Check sheet for the modelled part. Datum: model origin and axes. Units: mm. Face numbers are marked on the shaded views. A direction names the side the tool comes from. Round coordinates to 2 decimals unless told otherwise and drop trailing zeros. Write each loop counter-clockwise with the first axis right and the second up, starting at its lowest first coordinate (ties: lowest second). Pieces come first, ordered by that corner, then holes.
Item 1: Release check for a two-part mould opening along Y. For the marked faces 3, 4 and 5 record: +Y half, -Y half, draft (parallel to the pull), parting line (faces both ways), or undercut.
Item 2: Cross-section at C-C on x = 24. Enter the section's corners in (y, z), plus the area to 3 significant figures.
Item 3: Material ranges on line 1 (Z direction, x = 0, y = -1.7); line 2 (Y direction, x = 1, z = -26); line 3 (X direction, y = 11, z = -22.5), recorded low to high.
Item 4: Tool access check on the marked faces 1 and 2. Record the directions out of +Z, -Z, +X, -X, +Y, -Y that give a thin tool (end or side, any length) a straight path to the whole face; none if there is none.
Item 5: Cross-section at A-A on x = 0. Enter the section's corners in (y, z).
Item 6: Cross-section at D-D on z = -32.5. Enter the section's corners in (x, y).
Item 7: Cross-section at B-B on y = 13.5. Enter the section's corners in (x, z), plus the area to 3 significant figures.
Item 8: Go/stop test with flat-tipped pins: pin 1 Ø17.5 at (x, z) = (0, 0) entering from +Y; pin 2 Ø10 at (x, z) = (-9.5, 2) entering from +Y; pin 3 Ø8 at (x, y) = (-7.5, 16.5) entering from +Z; pin 4 Ø10 at (x, y) = (-20.5, 37.5) entering from +Z. Record where each tip stops, or that it passes through.
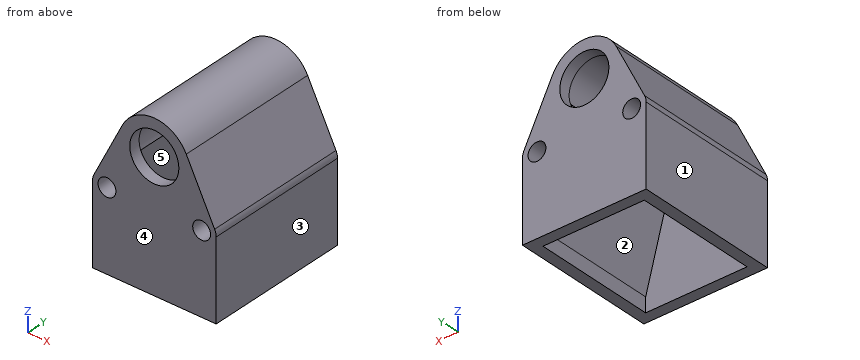
from build123d import *

# Parameters (mm, degrees)
SKETCH1_R           = 4
BOSS_EXTRUDE3_DEPTH = 55
SKETCH4_R           = 4
SKETCH4_R_2         = 11
BOSS_EXTRUDE4_DEPTH = 5
SKETCH5_R           = 11
SKETCH5_R_2         = 4
BOSS_EXTRUDE5_DEPTH = 5


with BuildPart() as part:
    # Sketch1 → Boss-Extrude3 (new body)
    with BuildSketch(Plane(origin=(0, 0, 0), x_dir=(1, 0, 0), z_dir=(0, 1, 0))):
        with BuildLine():
            Line((14.314144176, -7.14879546), (27.028324507, 18.30900528))
            ThreePointArc((27.028324507, 18.30900528), (27.539667178, 19.721272969), (27.713203436, 21.213203436))
            Line((27.713203436, 21.213203436), (27.713203436, 56.823174316))
            Line((27.713203436, 56.823174316), (22.713203436, 56.823174316))
            Line((22.713203436, 56.823174316), (22.713203436, 50.281094638))
            Line((22.713203436, 50.281094638), (10.285426583, 3.9))
            ThreePointArc((10.285426583, 3.9), (0, -11), (-10.285426583, 3.9))
            Line((-10.285426583, 3.9), (-22.713203436, 50.281094638))
            Line((-22.713203436, 50.281094638), (-22.713203436, 56.823174316))
            Line((-22.713203436, 56.823174316), (-27.713203436, 56.823174316))
            Line((-27.713203436, 56.823174316), (-27.713203436, 21.213203436))
            ThreePointArc((-27.713203436, 21.213203436), (-27.539667178, 19.721272969), (-27.028324507, 18.30900528))
            Line((-27.028324507, 18.30900528), (-14.314144176, -7.14879546))
            ThreePointArc((-14.314144176, -7.14879546), (0, -16), (14.314144176, -7.14879546))
        make_face()
        with Locations((-21.213203436, 21.213203436)):
            Circle(SKETCH1_R, mode=Mode.SUBTRACT)
        with Locations((21.213203436, 21.213203436)):
            Circle(SKETCH1_R, mode=Mode.SUBTRACT)
    extrude(amount=BOSS_EXTRUDE3_DEPTH)

    # Sketch4 → Boss-Extrude4 (add)
    with BuildSketch(Plane(origin=(0, 55, 0), x_dir=(1, 0, 0), z_dir=(0, 1, 0))):
        with BuildLine():
            Line((-27.713203436, 21.213203436), (-27.713203436, 56.823174316))
            Line((-27.713203436, 56.823174316), (27.713203436, 56.823174316))
            Line((27.713203436, 56.823174316), (27.713203436, 21.213203436))
            ThreePointArc((27.713203436, 21.213203436), (27.539667178, 19.721272969), (27.028324507, 18.30900528))
            Line((27.028324507, 18.30900528), (14.314144176, -7.14879546))
            ThreePointArc((14.314144176, -7.14879546), (0, -16), (-14.314144176, -7.14879546))
            Line((-14.314144176, -7.14879546), (-27.028324507, 18.30900528))
            ThreePointArc((-27.028324507, 18.30900528), (-27.539667178, 19.721272969), (-27.713203436, 21.213203436))
        make_face()
        with Locations((-21.213203436, 21.213203436)):
            Circle(SKETCH4_R, mode=Mode.SUBTRACT)
        with Locations((21.213203436, 21.213203436)):
            Circle(SKETCH4_R, mode=Mode.SUBTRACT)
        Circle(SKETCH4_R_2, mode=Mode.SUBTRACT)
    extrude(amount=BOSS_EXTRUDE4_DEPTH)

    # Sketch5 → Boss-Extrude5 (add)
    with BuildSketch(Plane.XZ):
        with BuildLine():
            Line((-27.028324507, -18.30900528), (-14.314144176, 7.14879546))
            ThreePointArc((-14.314144176, 7.14879546), (0, 16), (14.314144176, 7.14879546))
            Line((14.314144176, 7.14879546), (27.028324507, -18.30900528))
            ThreePointArc((27.028324507, -18.30900528), (27.539667178, -19.721272969), (27.713203436, -21.213203436))
            Line((27.713203436, -21.213203436), (27.713203436, -56.823174316))
            Line((27.713203436, -56.823174316), (-27.713203436, -56.823174316))
            Line((-27.713203436, -56.823174316), (-27.713203436, -21.213203436))
            ThreePointArc((-27.713203436, -21.213203436), (-27.539667178, -19.721272969), (-27.028324507, -18.30900528))
        make_face()
        Circle(SKETCH5_R, mode=Mode.SUBTRACT)
        with Locations((21.213203436, -21.213203436)):
            Circle(SKETCH5_R_2, mode=Mode.SUBTRACT)
        with Locations((-21.213203436, -21.213203436)):
            Circle(SKETCH5_R_2, mode=Mode.SUBTRACT)
    extrude(amount=BOSS_EXTRUDE5_DEPTH)


solid = part.part
Response values:
1. face 3: draft
1. face 4: -Y half
1. face 5: undercut
2. outline: (-5, -56.82) - (60, -56.82) - (60, -24.08) - (-5, -24.08) - close; (-5, -18.34) - (60, -18.34) - (60, -12.25) - (-5, -12.25) - close
2. area: 2,520 mm2
3. line 1: z = -56.82 to -11, 11 to 16
3. line 2: y = -5 to 0, 55 to 60
3. line 3: x = -27.71 to -25, -17.43 to -15.27, 15.27 to 17.43, 25 to 27.71
4. face 1: +Z, -Z, -X, +Y, -Y
4. face 2: -Z
5. outline: (-5, -56.82) - (0, -56.82) - (0, -11) - (-5, -11) - close; (-5, 11) - (60, 11) - (60, 16) - (-5, 16) - close; (55, -56.82) - (60, -56.82) - (60, -11) - (55, -11) - close
6. outline: (-27.71, -5) - (27.71, -5) - (27.71, 60) - (-27.71, 60) - close; hole (-17.95, 0) - (17.95, 0) - (17.95, 55) - (-17.95, 55) - close
7. outline: (-27.71, -56.82) - (-22.71, -56.82) - (-22.71, -50.28) - (-10.29, -3.9) arc R11 cw (long way) to (10.29, -3.9) - (22.71, -50.28) - (22.71, -56.82) - (27.71, -56.82) - (27.71, -21.21) arc R6.5 ccw to (27.03, -18.31) - (14.31, 7.15) arc R16 ccw to (-14.31, 7.15) - (-27.03, -18.31) arc R6.5 ccw to (-27.71, -21.21) - close; hole circle Ø8 at (-21.21, -21.21); hole circle Ø8 at (21.21, -21.21)
7. area: 1,160 mm2
8. pin 1: passes through
8. pin 2: stops at y = 60
8. pin 3: stops at z = 15.61
8. pin 4: stops at z = 4.77
